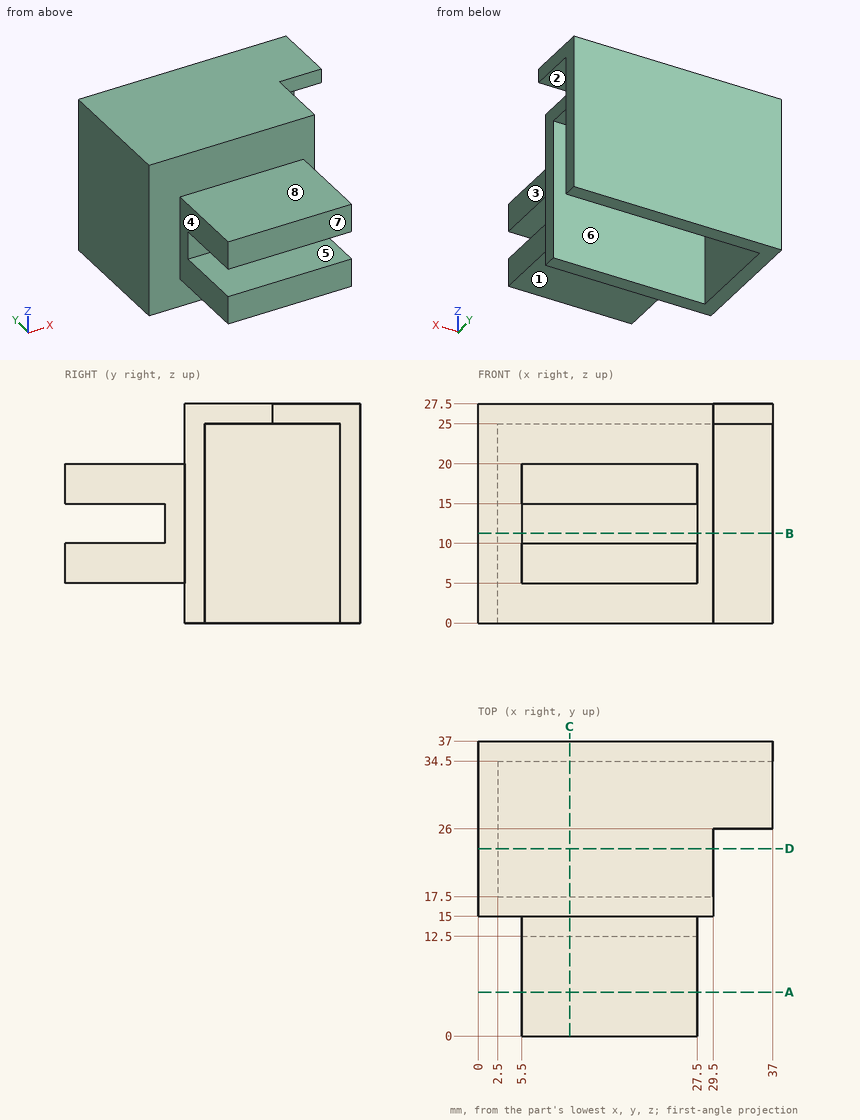
Geometry check sheet. Reference: drawing and pictorial views, mm from the part's lowest x, y, z. A direction names the side the tool comes from. Coordinates: 2 decimals unless noted, no trailing zeros. Order: outer loops, then holes, each group sorted by start corner. A loop starts at its lowest first (then second) coordinate and runs counter-clockwise, first axis right, second up. Notation, with made-up numbers: (26.25, 4) - (54.25, 4) arc R25 ccw to (54.25, 31) - close; hole circle Ø10 at (65.5, 81.25). An arc over 180 degrees is marked (long way). Answer in a Markdown table with one row per item. Add a question column.
1) Cross-section at B-B, the plane z = 11.25. Record the cut outline in (x, y).
2) Gauge pin test, flat ends, axial feed: P1, Ø16.5, axis at y = 6.5, z = 11, coming from the -X side; P2, Ø1, axis at y = 30.5, z = 5.5, coming from the -X side; P3, Ø12, axis at x = 13.5, y = 6, coming from the +Z side; P4, Ø4, axis at x = 6, y = 8, coming from the -Z side. Record the tip position at first contact, or that the pin passes through.
3) Material ranges on line 1 along Y through (x, z) = (28, 3.25); line 2 along Y through (x, z) = (20.5, 6.75); line 3 along Z through (x, y) = (7, 11), recorded low to high. Write a range as [from, to].
4) Set-up check for the marked faces 1, 2, 3, 4 and 5: record each of +Z, -Z, +X, -X, +Y, -Y from which the full face is reachable in a straight line by a thin tool's end or side.
5) Cross-section at C-C, the plane x = 11.5. Record the cut outline in (y, z), then the cut area to 4 significant figures.
6) Cross-section at A-A, the plane y = 5.5. Record the cut outline in (x, z).
7) Cross-section at D-D, the plane y = 23.5. Record the cut outline in (x, z), then the cut area to 3 significant figures.
8) Release check for a two-part mould opening along Y. For the marked faces 6, 7 and 8 record: +Y half, -Y half, draft (parallel to the pull), parting line (faces both ways), or undercut.
Check result:
| question | item | result |
|---|---|---|
| 1 | outline | (0, 15) - (5.5, 15) - (5.5, 12.5) - (27.5, 12.5) - (27.5, 15) - (29.5, 15) - (29.5, 17.5) - (2.5, 17.5) - (2.5, 34.5) - (37, 34.5) - (37, 37) - (0, 37) - close |
| 2 | P1 | stops at x = 5.5 |
| 2 | P2 | stops at x = 0 |
| 2 | P3 | stops at z = 20 |
| 2 | P4 | stops at z = 5 |
| 3 | line 1 | y = [15, 17.5], [34.5, 37] |
| 3 | line 2 | y = [0, 17.5], [34.5, 37] |
| 3 | line 3 | z = [5, 10], [15, 20] |
| 4 | face 1 | -Z, +X, -X, -Y |
| 4 | face 2 | -Z, +X |
| 4 | face 3 | +Z, -Z, +X, -Y |
| 4 | face 4 | +Z, -Z, -X, -Y |
| 4 | face 5 | +X, -X, -Y |
| 5 | outline | (0, 5) - (15, 5) - (15, 0) - (17.5, 0) - (17.5, 25) - (34.5, 25) - (34.5, 0) - (37, 0) - (37, 27.5) - (15, 27.5) - (15, 20) - (0, 20) - (0, 15) - (12.5, 15) - (12.5, 10) - (0, 10) - close |
| 5 | area | 342.5 mm² |
| 6 | outline | (5.5, 5) - (27.5, 5) - (27.5, 10) - (5.5, 10) - close; (5.5, 15) - (27.5, 15) - (27.5, 20) - (5.5, 20) - close |
| 7 | outline | (0, 0) - (2.5, 0) - (2.5, 25) - (29.5, 25) - (29.5, 27.5) - (0, 27.5) - close |
| 7 | area | 136 mm² |
| 8 | face 6 | undercut |
| 8 | face 7 | -Y half |
| 8 | face 8 | draft |
